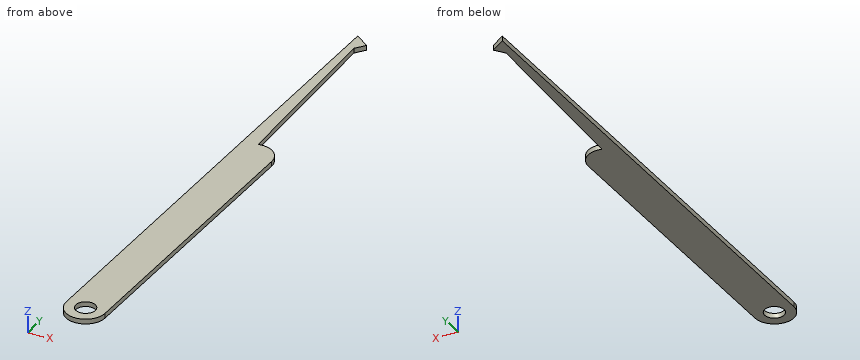
Solid Edge part; units mm, degrees
sketch "Sketch1" plane through (0, 0, 0) normal (0, 0, 1) x (1, 0, 0)
  line L0 (4, -30) -> (4, 30)
  arc A0 (4, 30) -> (-1, 33.873) centre (0, 30) ccw
  line L1 (-2.5, 71) -> (-1, 33.873)
  line L2 (-1, 73) -> (-2.5, 71)
  line L3 (-4, 75) -> (-1, 73)
  line L4 (-4, 30) -> (-4, 75)
  line L5 (-4, 30) -> (-4, -30)
  arc A1 (-4, -30) -> (4, -30) centre (0, -30) ccw
  dimension "D1" = 4
  dimension "D2" = 2.5
extrude "Ajout_matière_1" add sketch "Sketch1" along normal blind 1
sketch "Sketch2" plane through (0, 0, 0) normal (0, 0, 1) x (1, 0, 0)
  circle A0 centre (0, -30) radius 2
extrude "Cutout1" cut sketch "Sketch2" along normal up to next
properties material "Acier S235"
Design review of the part built by this model. Coordinates are the model's own, in mm. Round coordinates to 2 decimals unless told otherwise and drop trailing zeros. Write each loop counter-clockwise with the first axis right and the second up, starting at its lowest first coordinate (ties: lowest second). Pieces come first, ordered by that corner, then holes. Notation, with made-up numbers: (-31.5, 9) - (24.5, 9) arc R28 cw to (24.5, 27) - close; hole circle Ø7 at (-24.5, 87). An arc over 180 degrees is marked (long way). Return JSON: item names as keys, results as strings. Group by question number.
Item 1: We need section A-A on x = 0. Write out the cut boundary in (y, z).
Item 2: We need section C-C on y = 44.5. Write out the cut boundary in (x, z).
Item 3: For probe 1 along X at (y, z) = (-30, 0.25); probe 2 along Y at (x, z) = (0, 0.3); probe 3 along Y at (x, z) = (0.75, 0.35), list the stretches that pass through material, from the lowest coordinate up. Write a range as [from, to].
Item 4: We need section B-B on z = 0.8. Write out the cut boundary in (x, y), and give its area (3 significant figures).
Item 5: Insertion check: P1, Ø2.5, axis at x = 0, y = -30, coming from the -Z side. The pin has a flat end and moves straight along its axis. Give the tip position at first contact, or say it passes through.
Model answer:
{
 "1": {"outline": "(-34, 0) - (-32, 0) - (-32, 1) - (-34, 1) - close; (-28, 0) - (34, 0) - (34, 1) - (-28, 1) - close"},
 "2": {"outline": "(-4, 0) - (-1.43, 0) - (-1.43, 1) - (-4, 1) - close"},
 "3": {"probe 1": "x = [-4, -2], [2, 4]", "probe 2": "y = [-34, -32], [-28, 34]", "probe 3": "y = [-33.93, -31.85], [-28.15, 33.93]"},
 "4": {"outline": "(-4, -30) arc R4 ccw to (4, -30) - (4, 30) arc R4 ccw to (-1, 33.87) - (-2.5, 71) - (-1, 73) - (-4, 75) - close; hole circle Ø4 at (0, -30)", "area": "612 mm²"},
 "5": {"P1": "passes through"}
}
